```python
from build123d import *

# Parameters (mm, degrees)
F0_W     = 80
F0_H     = 80
F0_R     = 13
F1_DEPTH = 20
F2_R     = 16
F2_R_2   = 13
F3_DEPTH = 9
F4_R     = 3
F5_DEPTH = 20
F6_R     = 3
F7_DEPTH = 20


with BuildPart() as f1:
    # F0 (on Front) → F1 (new body)
    with BuildSketch(Plane.XZ):
        with Locations((40, 40)):
            Rectangle(F0_W, F0_H)
        with Locations((40, 40)):
            Circle(F0_R, mode=Mode.SUBTRACT)
    extrude(amount=F1_DEPTH)

    # F2 (on face) → F3 (cut)
    with BuildSketch(Plane(origin=(0, 0, 0), x_dir=(-1, 0, 0), z_dir=(0, 1, 0))):
        with Locations((-40, 40)):
            Circle(F2_R)
        with Locations((-40, 40)):
            Circle(F2_R_2, mode=Mode.SUBTRACT)
    extrude(amount=-F3_DEPTH, mode=Mode.SUBTRACT)

    # F4 (on face) → F5 (cut)
    with BuildSketch(Plane.YZ.offset(80)):
        with Locations((-10, 65)):
            Circle(F4_R)
        with Locations((-10, 15)):
            Circle(F4_R)
    extrude(amount=-F5_DEPTH, mode=Mode.SUBTRACT)

    # F6 (on face) → F7 (cut)
    with BuildSketch(Plane(origin=(0, 0, 0), x_dir=(0, -1, 0), z_dir=(-1, 0, 0))):
        with Locations((10, 65)):
            Circle(F6_R)
        with Locations((10, 15)):
            Circle(F6_R)
    extrude(amount=-F7_DEPTH, mode=Mode.SUBTRACT)


solid = f1.part
```
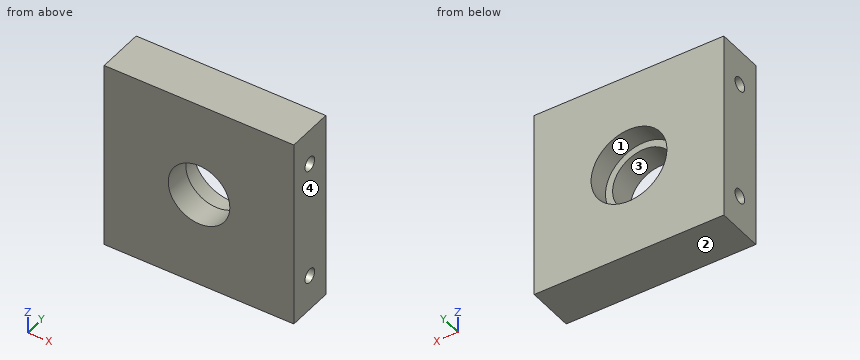
CAD build for the part. Positions are in the model's coordinates, mm. Face numbers are marked on the shaded views. Round coordinates to 2 decimals unless told otherwise and drop trailing zeros. Write each loop counter-clockwise with the first axis right and the second up, starting at its lowest first coordinate (ties: lowest second). Pieces come first, ordered by that corner, then holes. Notation, with made-up numbers: (-27.75, 87) -> (13.25, 87) arc R29 cw to (13.25, 125) -> close; hole circle Ø8 at (59, 16.25). An arc over 180 degrees is marked (long way). Answer in a Markdown table with one row per item. Add a question column.
Item 1: Drop flat-ended pins along their axis: pin 1 Ø16 at (x, z) = (39.5, 33) entering from +Y; pin 2 Ø3 at (y, z) = (-9, 64.5) entering from -X; pin 3 Ø5.5 at (y, z) = (-10, 65) entering from +X. Give the stop position or say it passes through.
Item 2: Saw through at D-D, the plane z = 15. Write the cut outline in (x, y).
Item 3: Mould opens along Z. For the marked faces 1, 2, 3 and 4 say: pulls with the +Z half, pulls with the -Z half, needs draft (parallel to the pull), parting line crosses it, or undercut.
Item 4: Saw through at A-A, the plane z = 40. Write the cut outline in (x, y).
Item 5: Saw through at C-C, the plane y = -4.75. Write the cut outline in (x, z).
Item 6: Drill centre lines: line 1 (Z direction, x = 13, y = -10); line 2 (Z direction, x = 40.5, y = -7.25); line 3 (Z direction, x = 40, y = -13). Where is each one in solid material? Low to high. Write a range as from..to.
Item 7: Saw through at B-B, the plane x = 40. Write the cut outline in (y, z), then the cut area to 3 significant figures.
Findings below:
| question | item | result |
|---|---|---|
| 1 | pin 1 | stops at y = -9 |
| 1 | pin 2 | stops at x = 20 |
| 1 | pin 3 | stops at x = 60 |
| 2 | outline | (0, -20) -> (80, -20) -> (80, -13) -> (60, -13) -> (60, -7) -> (80, -7) -> (80, 0) -> (0, 0) -> (0, -7) -> (20, -7) -> (20, -13) -> (0, -13) -> close |
| 3 | face 1 | undercut |
| 3 | face 2 | pulls with the -Z half |
| 3 | face 3 | undercut |
| 3 | face 4 | needs draft |
| 4 | outline | (0, -20) -> (27, -20) -> (27, -9) -> (24, -9) -> (24, 0) -> (0, 0) -> close; (53, -20) -> (80, -20) -> (80, 0) -> (56, 0) -> (56, -9) -> (53, -9) -> close |
| 5 | outline | (0, 0) -> (80, 0) -> (80, 80) -> (0, 80) -> close; hole circle Ø32 at (40, 40) |
| 6 | line 1 | z = 0..12, 18..62, 68..80 |
| 6 | line 2 | z = 0..24.01, 55.99..80 |
| 6 | line 3 | z = 0..27, 53..80 |
| 7 | outline | (-20, 0) -> (0, 0) -> (0, 24) -> (-9, 24) -> (-9, 27) -> (-20, 27) -> close; (-20, 53) -> (-9, 53) -> (-9, 56) -> (0, 56) -> (0, 80) -> (-20, 80) -> close |
| 7 | area | 1,030 mm^2 |
